```python
from build123d import *

# Parameters (mm, degrees)
F1_DEPTH = 32
F4_DEPTH = 55
F5_R     = 4.99999


# Not quite as in the source:
# - a fillet or chamfer is up to 0.001 mm smaller than in the source, because OpenCascade refuses the exact size


with BuildPart() as f1:
    # F0 (on Front) → F1 (new body)
    with BuildSketch(Plane.XZ):
        Polygon((0, 46), (0, 0), (50, 0), (50, 40), align=None)
    extrude(amount=-F1_DEPTH)

    # F3 (on face) → F4 (cut, symmetric)
    with BuildSketch(Plane(origin=(44.5961827524, 0, -5.3177728391), x_dir=(0, 1, 0), z_dir=(0.9929655081, 0, -0.1184039683))):
        with BuildLine():
            Line((5, 47.6340688765), (5, 35.6388187396))
            ThreePointArc((5, 35.6388187396), (16, 24.6388187396), (27, 35.6388187396))
            Line((27, 35.6388187396), (27, 47.6340688765))
            Line((27, 47.6340688765), (5, 47.6340688765))
        make_face()
    extrude(amount=F4_DEPTH, both=True, mode=Mode.SUBTRACT)

    # F5 (radius 5 in the source; OpenCascade refuses exactly that, so slightly less here)
    f5_edges = [f1.edges().sort_by_distance(p)[0] for p in [
        (25, 27, 43),
        (25, 5, 43),
    ]]
    fillet(f5_edges, radius=F5_R)


solid = f1.part
```
Input: part model. Units: mm. Frame: model coordinates. A direction names the side the tool comes from. Coordinates: 2 decimals unless noted, no trailing zeros. Write each loop counter-clockwise with the first axis right and the second up, starting at its lowest first coordinate (ties: lowest second). Pieces come first, ordered by that corner, then holes.
1) Section B-B on y = 3.5. Output: boundary loops of the cut face in (x, z).
2) Set-up query: faces 4 (the flat face through (0, 16, 18)), 5 (the cylindrical face through (24.77, 28.5, 41.59)). Return all of +Z, -Z, +X, -X, +Y, -Y with unobstructed straight access to the full face (end or side cutting, diameter ignored); none if empty.
3) Mould query, pull axis Y, two halves, no side actions, for faces 1 (the flat face through (25, 0, 23)), 2 (the flat face through (25, 32, 23)), 3 (the cylindrical face through (24.71, 15.76, 21.87)). Classes: pulls with the +Y half, pulls with the -Y half, needs draft (parallel to the pull), parting line crosses it, or undercut.
4) Section A-A on y = 9. Output: boundary loops of the cut face in (x, z).
5) Material intervals for line 1 along Y through (x, z) = (20, 27); line 2 along Z through (x, y) = (48, 8); line 3 along Z through (x, y) = (17, 7.5), sorted ascending.
Check result:
1. outline: (0, 0) - (50, 0) - (50, 38.56) - (0, 44.56) - close
2. face 4: +Z, -Z, -X, +Y, -Y
2. face 5: +Z, +X
3. face 1: pulls with the -Y half
3. face 2: pulls with the +Y half
3. face 3: undercut
4. outline: (0, 0) - (50, 0) - (50, 21.38) - (0, 27.35) - close
5. line 1: y = 0 to 7.1, 24.9 to 32
5. line 2: z = 0 to 22.56
5. line 3: z = 0 to 26.83
